from build123d import *

# Parameters (mm, degrees)
F0_W     = 101.6
F0_H     = 76.2
F1_DEPTH = 19.05
F2_W     = 50.8
F2_H     = 38.1
F3_DEPTH = 25.4
F4_R     = 5.08


with BuildPart() as f1:
    # F0 (on Top) → F1 (new body)
    with BuildSketch(Plane.XY):
        Rectangle(F0_W, F0_H)
    extrude(amount=F1_DEPTH)

    # F2 (on face) → F3 (cut)
    with BuildSketch(Plane.XY.offset(19.05)):
        Rectangle(F2_W, F2_H)
    extrude(amount=-F3_DEPTH, mode=Mode.SUBTRACT)

    # F4
    f4_edges = [f1.edges().sort_by_distance(p)[0] for p in [
        (-50.8, 38.1, 9.525),
        (-50.8, -38.1, 9.525),
        (50.8, 38.1, 9.525),
        (25.4, -19.05, 9.525),
        (-25.4, 19.05, 9.525),
        (50.8, -38.1, 9.525),
        (-25.4, -19.05, 9.525),
        (-25.4, 0, 19.05),
        (-50.8, 0, 19.05),
        (0, -38.1, 19.05),
        (50.8, 0, 19.05),
        (0, 38.1, 19.05),
        (25.4, 19.05, 9.525),
        (0, -19.05, 19.05),
        (25.4, 0, 19.05),
        (0, 19.05, 19.05),
    ]]
    fillet(f4_edges, radius=F4_R)


solid = f1.part
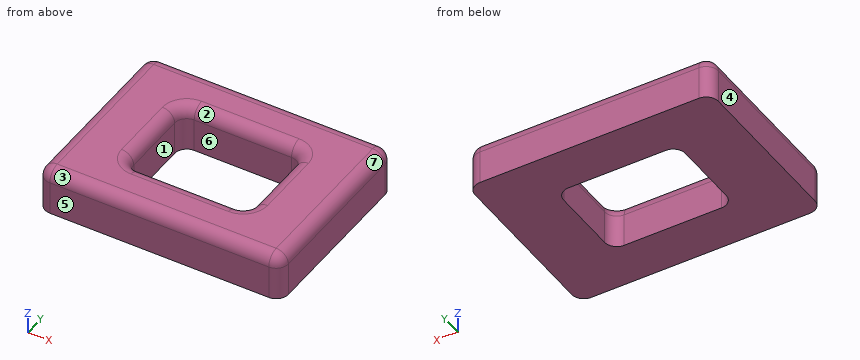
Can you work these out from the model? Positions are in its coordinate system, mm. Face numbers are marked on the shaded views. A direction names the side the tool comes from. Coordinates: 2 decimals unless noted, no trailing zeros. Write each loop counter-clockwise with the first axis right and the second up, starting at its lowest first coordinate (ties: lowest second). Pieces come first, ordered by that corner, then holes. Notation, with made-up numbers: M 16,59 L 29,59 A21 ccw 29,86 Z; hole C 17.5,32 d8. An arc over 180 degrees is marked long. Use one line per item in the form item = value.
Q1. I need wall thicknesses on line 1 along X through (y, z) = (-5, 7.75); line 2 along Y through (x, z) = (-15, 5.5). Which ranges of each line are inside material? Lowest first, please. Write a range as from..to.
Model answer:
line_1 = -50.8..-25.4, 25.4..50.8
line_2 = -38.1..-19.05, 19.05..38.1
Q2. If we section it at A-A (x = 19): Write out the boundary of the cut face in (y, z).
Model answer:
outline = M -38.1,0 L -19.05,0 L -19.05,13.97 A5.08 ccw -24.13,19.05 L -33.02,19.05 A5.08 ccw -38.1,13.97 Z; M 19.05,0 L 38.1,0 L 38.1,13.97 A5.08 ccw 33.02,19.05 L 24.13,19.05 A5.08 ccw 19.05,13.97 Z
Q3. If we section it at B-B (y = -6.5): Write out the boundary of the cut face in (x, z).
Model answer:
outline = M -50.8,0 L -25.4,0 L -25.4,13.97 A5.08 ccw -30.48,19.05 L -45.72,19.05 A5.08 ccw -50.8,13.97 Z; M 25.4,0 L 50.8,0 L 50.8,13.97 A5.08 ccw 45.72,19.05 L 30.48,19.05 A5.08 ccw 25.4,13.97 Z
Q4. If we section it at C-C (z = 2.5): Write out the boundary of the cut face in (x, y), then the cut area to 3 significant figures.
Model answer:
outline = M -50.8,-33.02 A5.08 ccw -45.72,-38.1 L 45.72,-38.1 A5.08 ccw 50.8,-33.02 L 50.8,33.02 A5.08 ccw 45.72,38.1 L -45.72,38.1 A5.08 ccw -50.8,33.02 Z; hole M -25.4,-13.97 A5.08 ccw -20.32,-19.05 L 20.32,-19.05 A5.08 ccw 25.4,-13.97 L 25.4,13.97 A5.08 ccw 20.32,19.05 L -20.32,19.05 A5.08 ccw -25.4,13.97 Z
area = 5,810 mm^2
Q5. For P1, Ø1.5, axis at x = 30, y = -22.5, coming from the -Z side, with a flat end and sliding along its axis, tell me the tip position at first contact or that it passes through.
Model answer:
P1 = 0
Q6. If we section it at D-D (z = 17.75): Write out the boundary of the cut face in (x, y).
Model answer:
outline = M -49.11,-33.02 A3.39 ccw -45.72,-36.41 L 45.72,-36.41 A3.39 ccw 49.11,-33.02 L 49.11,33.02 A3.39 ccw 45.72,36.41 L -45.72,36.41 A3.39 ccw -49.11,33.02 Z; hole M -27.09,-13.97 A6.77 ccw -20.32,-20.74 L 20.32,-20.74 A6.77 ccw 27.09,-13.97 L 27.09,13.97 A6.77 ccw 20.32,20.74 L -20.32,20.74 A6.77 ccw -27.09,13.97 Z
Q7. For the marked faces 1, 2 and 3, which set-ups out of +Z, -Z, +X, -X, +Y, -Y let a thin tool reach every point of the face, with its end or its side?
Model answer:
face_1 = +Z, -Z
face_2 = +Z
face_3 = +Z, +X, -X, -Y
Q8. We'd pull the mould along X, two halves only. Please class the marked faces 4, 5, 6 and 7: +X half, -X half, draft (parallel to the pull), parting line (faces both ways), or undercut.
Model answer:
face_4 = -X half
face_5 = draft
face_6 = undercut
face_7 = +X half
